Read the model definition and answer for the solid it produces. Units are mm, in the model's axes. Face numbers are marked on the shaded views. A direction names the side the tool comes from. Coordinates: 2 decimals unless noted, no trailing zeros. Loops run counter-clockwise (first coordinate to the right, second up) from the corner with the lowest first, then second, coordinate; pieces in that order, holes last. Notation, with made-up numbers: (61.25, 1) - (84.25, 1) arc R18 cw to (84.25, 13) - close; hole circle Ø9 at (15.25, -18). An arc over 180 degrees is marked (long way). Use CSV: the item, a comma, the result in double quotes.
```python
from build123d import *

# Parameters (mm, degrees)
BOSS_EXTRUDE1_DEPTH     = 10.3
SKETCH2_OUTSIDE_W       = 43.282
SKETCH2_OUTSIDE_H       = 43.282
CUT_EXTRUDE1_DEPTH      = 5
CUT_EXTRUDE2_DEPTH      = 24.239836488
CUT_EXTRUDE2_DEPTH_BACK = 24.239836488
SKETCH4_R               = 1
CUT_EXTRUDE3_DEPTH      = 38.230229653
CUT_EXTRUDE3_DEPTH_BACK = 38.230229653
SKETCH6_W               = 12
SKETCH6_H               = 22
CUT_EXTRUDE4_DEPTH      = 3.3


with BuildPart() as part:
    # Sketch1 → Boss-Extrude1 (new body)
    with BuildSketch(Plane(origin=(0, 0, 0), x_dir=(1, 0, 0), z_dir=(0, 1, 0))):
        with BuildLine():
            Line((-13.5, 16), (13.5, 16))
            ThreePointArc((13.5, 16), (15.267766953, 15.267766953), (16, 13.5))
            Line((16, 13.5), (16, -13.5))
            ThreePointArc((16, -13.5), (15.267766953, -15.267766953), (13.5, -16))
            Line((13.5, -16), (-13.5, -16))
            ThreePointArc((-13.5, -16), (-15.267766953, -15.267766953), (-16, -13.5))
            Line((-16, -13.5), (-16, 13.5))
            ThreePointArc((-16, 13.5), (-15.267766953, 15.267766953), (-13.5, 16))
        make_face()
    extrude(amount=BOSS_EXTRUDE1_DEPTH)

    # Sketch2 outside → Cut-Extrude1 (cut)
    with BuildSketch(Plane(origin=(0, 10.3, 0), x_dir=(1, 0, 0), z_dir=(0, 1, 0))):
        Rectangle(SKETCH2_OUTSIDE_W, SKETCH2_OUTSIDE_H)
        with BuildLine():
            Line((-9.5, -12), (9.5, -12))
            ThreePointArc((9.5, -12), (11.267766953, -11.267766953), (12, -9.5))
            Line((12, -9.5), (12, 9.5))
            ThreePointArc((12, 9.5), (11.267766953, 11.267766953), (9.5, 12))
            Line((9.5, 12), (-9.5, 12))
            ThreePointArc((-9.5, 12), (-11.267766953, 11.267766953), (-12, 9.5))
            Line((-12, 9.5), (-12, -9.5))
            ThreePointArc((-12, -9.5), (-11.267766953, -11.267766953), (-9.5, -12))
        make_face(mode=Mode.SUBTRACT)
    extrude(amount=-CUT_EXTRUDE1_DEPTH, mode=Mode.SUBTRACT)

    # Sketch4 → Cut-Extrude2 (cut, two sides: drawn at the far end of the back side and taken through both)
    with BuildSketch(Plane(origin=(0, 5.3, 0), x_dir=(1, 0, 0), z_dir=(0, 1, 0)).offset(-CUT_EXTRUDE2_DEPTH_BACK)):
        with Locations(Location((-13.5, 13.5, 0), (0, 0, 270))):
            Circle(SKETCH4_R)
        with Locations(Location((13.5, -13.5, 0), (0, 0, 270))):
            Circle(SKETCH4_R)
        with Locations(Location((-13.5, -13.5, 0), (0, 0, 270))):
            Circle(SKETCH4_R)
        with Locations(Location((13.5, 13.5, 0), (0, 0, 270))):
            Circle(SKETCH4_R)
    extrude(amount=CUT_EXTRUDE2_DEPTH + CUT_EXTRUDE2_DEPTH_BACK, mode=Mode.SUBTRACT)

    # Sketch5 → Cut-Extrude3 (cut, two sides: drawn at the far end of the back side and taken through both)
    with BuildSketch(Plane.XY.offset(16).offset(-CUT_EXTRUDE3_DEPTH_BACK)):
        Polygon((-17.244345891, 3.3), (-17.244345891, -0.614628683), (-6, -0.614628683), (-6, 0), (-6, 0.3), (-6, 3.3), align=None)
        Polygon((6, 3.3), (6, 0.3), (6, 0), (6, -0.614628683), (18.655939846, -0.614628683), (18.655939846, 3.3), align=None)
    extrude(amount=CUT_EXTRUDE3_DEPTH + CUT_EXTRUDE3_DEPTH_BACK, mode=Mode.SUBTRACT)

    # Sketch6 → Cut-Extrude4 (cut)
    with BuildSketch(Plane.XZ):
        Rectangle(SKETCH6_W, SKETCH6_H)
    extrude(amount=-CUT_EXTRUDE4_DEPTH, mode=Mode.SUBTRACT)


solid = part.part
```
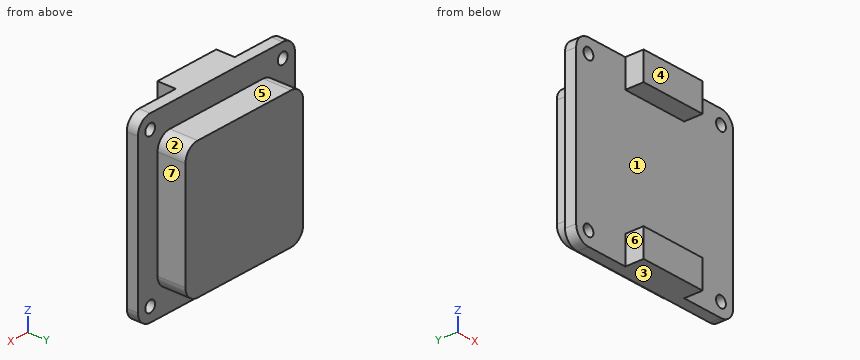
Q1. Given P1, Ø6, axis at x = -3.5, y = 7.5, coming from the -Z side; P2, Ø1, axis at x = -10, z = -12, coming from the -Y side; P3, Ø1, axis at y = 1, z = -13, coming from the +X side; P4, Ø3, axis at x = -13.5, z = 13.5, coming from the +Y side, each flat-ended and moving along its own axis, determine where each tip first touches the part or whether it passes through.
Reported:
P1,"stops at z = -16"
P2,"stops at y = 3.3"
P3,"stops at x = 6"
P4,"stops at y = 5.3"
Q2. The part is cut by section C-C on z = 14. Determine the outline of the cut face in (x, y), and give its area (3 significant figures).
Reported:
outline,"(-15.95, 3.3) - (-14.37, 3.3) - (-14.37, 5.3) - (-15.95, 5.3) - close; (-12.63, 3.3) - (-6, 3.3) - (-6, 0) - (6, 0) - (6, 3.3) - (12.63, 3.3) - (12.63, 5.3) - (-12.63, 5.3) - close; (14.37, 3.3) - (15.95, 3.3) - (15.95, 5.3) - (14.37, 5.3) - close"
area,"96.5 mm²"
Q3. The part is cut by section D-D on z = -11.5. Determine the outline of the cut face in (x, y), and give its area (3 significant figures).
Reported:
outline,"(-16, 3.3) - (-6, 3.3) - (-6, 0) - (6, 0) - (6, 3.3) - (16, 3.3) - (16, 5.3) - (11, 5.3) - (11, 10.3) - (-11, 10.3) - (-11, 5.3) - (-16, 5.3) - close"
area,"214 mm²"
Q4. The part is cut by section B-B on x = -1.5. Determine the outline of the cut face in (y, z).
Reported:
outline,"(0, -16) - (5.3, -16) - (5.3, -12) - (10.3, -12) - (10.3, 12) - (5.3, 12) - (5.3, 16) - (0, 16) - (0, 11) - (3.3, 11) - (3.3, -11) - (0, -11) - close"
Q5. The part is cut by section A-A on y = 1.25. Determine the outline of the cut face in (x, z).
Reported:
outline,"(-6, -16) - (6, -16) - (6, -11) - (-6, -11) - close; (-6, 11) - (6, 11) - (6, 16) - (-6, 16) - close"
Q6. For a pull along Z with two mould halves and no side action, classify the marked faces 1, 2, 3 and 4 as +Z half, -Z half, draft (parallel to the pull), parting line (faces both ways), or undercut.
Reported:
face 1,"undercut"
face 2,"+Z half"
face 3,"-Z half"
face 4,"draft"
Q7. Find the intervals of material crossed by probe 1 along X at (y, z) = (4.3, -13.5); probe 2 along Y at (x, z) = (13, 8), in increasing order. Write a range as [from, to].
Reported:
probe 1,"x = [-16, -14.5], [-12.5, 12.5], [14.5, 16]"
probe 2,"y = [3.3, 5.3]"
Q8. A tool of negligible diameter and unlimited length cuts with its end or side. For the marked faces 5, 6 and 7, from which of +Z, -Z, +X, -X, +Y, -Y can it reach the whole face along a straight path? Write none if from no direction.
Reported:
face 5,"+Z, +X, -X, +Y"
face 6,"+Z, -Z, -X, -Y"
face 7,"+Z, -Z, +X, +Y"
